Part model, mm, in its own coordinate system. Round coordinates to 2 decimals unless told otherwise and drop trailing zeros. Write each loop counter-clockwise with the first axis right and the second up, starting at its lowest first coordinate (ties: lowest second). Pieces come first, ordered by that corner, then holes.
1) Drill centre lines: L1, parallel to X at y = -15.5, z = -0.5; L2, parallel to Y at x = -8, z = -5.25; L3, parallel to Y at x = 3, z = -0.5. Where is each one in solid material? Low to high.
2) Saw through at A-A on x = 28.5. Write the cut outline in (y, z), and give its area (3 significant figures).
3) Flat gauge pin, fed straight in: pin 1 (1.5 mm diameter, centred on y = 31.5, z = -1.5, fed in from -X). Where does the tip first touch, or does it go through?
```python
from build123d import *

# Parameters (mm, degrees)
F1_DEPTH = 3
F1_TAPER = -30


with BuildPart() as f1:
    # F0 (on Top) → F1 (new body)
    with BuildSketch(Plane.XY):
        Polygon((36.0686861882, -19.9420294206), (18.0343430941, 11.2943690995), (0, -19.9420294206), align=None)
        Polygon((0, -19.9420294206), (-18.0343430941, 11.2943690995), (-36.0686861882, -19.9420294206), align=None)
        Polygon((18.0343430941, 11.2943690995), (0, 42.5307676196), (-18.0343430941, 11.2943690995), align=None)
    extrude(amount=-F1_DEPTH, taper=F1_TAPER)

    # F2: union 

    # F3: F1 across face


with BuildPart() as f1_1:
    add(f1.part)
    add(f1.part.mirror(Plane(origin=(0, 0.8822362595, -3), x_dir=(1, 0, 0), z_dir=(0, 0, -1))))


solid = f1_1.part
```
Completed:
1. L1: x = -33.84 to -2.23, 2.23 to 33.84
1. L2: y = -20.38 to -5.22, 10.86 to 29.54
1. L3: y = -20.23 to -14.17, 11.01 to 37.91
2. outline: (-21.67, -3) - (-19.94, -6) - (-6.83, -6) - (-3.37, -3) - (-6.83, 0) - (-19.94, 0) - close
2. area: 94.2 mm2
3. pin 1: stops at x = -8.03
